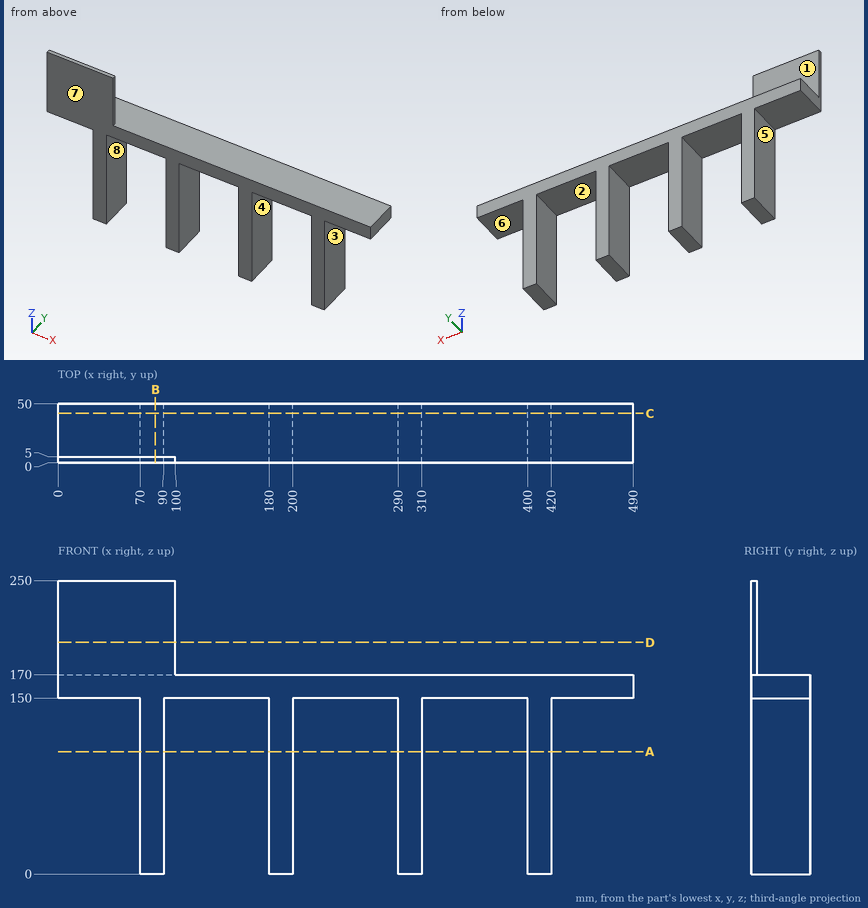
Answer from the drawing. Dimensions are ordinates in mm from the lowest x, y and z of the part. A direction names the side the tool comes from. Coordinates: 2 decimals unless noted, no trailing zeros. Loops run counter-clockwise (first coordinate to the right, second up) from the corner with the lowest first, then second, coordinate; pieces in that order, holes last. Notation, with made-up numbers: (61.5, -29) -> (83.5, -29) arc R19 ccw to (83.5, -6) -> close; hole circle Ø10 at (31.5, -12). An arc over 180 degrees is marked (long way). Answer in a Markdown table with one row per item.
Item 1: Each of these flat-tipped pins is pushed along its axis until it touches: P1, Ø5, axis at x = 286.5, y = 5.5, coming from the +Z side; P2, Ø25, axis at y = 24.5, z = 87.5, coming from the +X side; P3, Ø25, axis at x = 445, y = 20, coming from the -Z side. Where does it stop, or does it pass through?
Returned:
| item | result |
|---|---|
| P1 | stops at z = 170 |
| P2 | stops at x = 420 |
| P3 | stops at z = 150 |
Item 2: A cutting plane is placed at A-A on z = 104.5. Determine the outline of the cut face in (x, y).
Returned:
| item | result |
|---|---|
| outline | (70, 0) -> (90, 0) -> (90, 50) -> (70, 50) -> close; (180, 0) -> (200, 0) -> (200, 50) -> (180, 50) -> close; (290, 0) -> (310, 0) -> (310, 50) -> (290, 50) -> close; (400, 0) -> (420, 0) -> (420, 50) -> (400, 50) -> close |
Item 3: Straight lines are drawn through the part: line 1 along X through (y, z) = (19, 132); line 2 along Z through (x, y) = (67, 24.5); line 3 along Z through (x, y) = (419, 40). For each, find the intervals that lie inside material, in ascending order. Write a range as [from, to].
Returned:
| item | result |
|---|---|
| line 1 | x = [70, 90], [180, 200], [290, 310], [400, 420] |
| line 2 | z = [150, 170] |
| line 3 | z = [0, 170] |
Item 4: For the marked faces 5, 6, 7 and 8, determine the directions among +Z, -Z, +X, -X, +Y, -Y from which every point of the face is accessible in a straight line to the end or side of a thin tool.
Returned:
| item | result |
|---|---|
| face 5 | -Z, -X, +Y, -Y |
| face 6 | -Z, +X, +Y, -Y |
| face 7 | +Z, -Z, +X, -X, -Y |
| face 8 | -Z, +Y, -Y |
Item 5: A cutting plane is placed at C-C on y = 42. Determine the outline of the cut face in (x, z), plus the area to 3 significant figures.
Returned:
| item | result |
|---|---|
| outline | (0, 150) -> (70, 150) -> (70, 0) -> (90, 0) -> (90, 150) -> (180, 150) -> (180, 0) -> (200, 0) -> (200, 150) -> (290, 150) -> (290, 0) -> (310, 0) -> (310, 150) -> (400, 150) -> (400, 0) -> (420, 0) -> (420, 150) -> (490, 150) -> (490, 170) -> (0, 170) -> close |
| area | 21,800 mm^2 |
Item 6: A cutting plane is placed at D-D on z = 197.5. Determine the outline of the cut face in (x, y).
Returned:
| item | result |
|---|---|
| outline | (0, 0) -> (100, 0) -> (100, 5) -> (0, 5) -> close |
Item 7: A cutting plane is placed at B-B on x = 83. Determine the outline of the cut face in (y, z), plus the area to 3 significant figures.
Returned:
| item | result |
|---|---|
| outline | (0, 0) -> (50, 0) -> (50, 170) -> (5, 170) -> (5, 250) -> (0, 250) -> close |
| area | 8,900 mm^2 |
Item 8: For a pull along X with two mould halves and no side action, classify the marked faces 1, 2, 3 and 4 as released by +X, released by -X, zero draft, split by the parting line, or undercut.
Returned:
| item | result |
|---|---|
| face 1 | zero draft |
| face 2 | undercut |
| face 3 | released by +X |
| face 4 | undercut |
